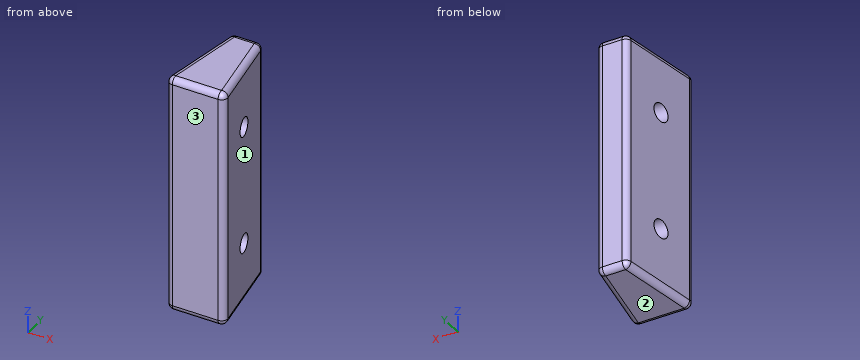
```python
from build123d import *

# Parameters (mm, degrees)
BOSS_EXTRUDE1_DEPTH     = 50.8
FILLET1_R               = 2.54
SKETCH4_R               = 3.96875
CUT_EXTRUDE1_DEPTH      = 13.241630529
CUT_EXTRUDE1_DEPTH_BACK = 13.241630529


with BuildPart() as part:
    # Sketch3 → Boss-Extrude1 (new body, symmetric)
    with BuildSketch(Plane.XY):
        Polygon((-12.7, 0), (12.7, 0), (6.35, 38.1), (-6.35, 38.1), align=None)
    extrude(amount=BOSS_EXTRUDE1_DEPTH, both=True)

    # Fillet1
    fillet1_edges = [part.edges().sort_by_distance(p)[0] for p in [
        (0, 0, 50.8),
        (9.525, 19.05, 50.8),
        (0, 38.1, 50.8),
        (9.525, 19.05, -50.8),
        (0, 0, -50.8),
        (-9.525, 19.05, -50.8),
        (0, 38.1, -50.8),
        (-9.525, 19.05, 50.8),
        (6.35, 38.1, 0),
        (12.7, 0, 0),
        (-12.7, 0, 0),
        (-6.35, 38.1, 0),
    ]]
    fillet(fillet1_edges, radius=FILLET1_R)

    # Sketch4 → Cut-Extrude1 (cut, two sides)
    with BuildSketch(Plane(origin=(0, 0, 0), x_dir=(0, 0, -1), z_dir=(1, 0, 0))) as cut_extrude1_sk:
        with Locations((-25.4, 19.05)):
            Circle(SKETCH4_R)
        with Locations((25.4, 19.05)):
            Circle(SKETCH4_R)
    extrude(amount=CUT_EXTRUDE1_DEPTH, mode=Mode.SUBTRACT)
    extrude(cut_extrude1_sk.sketch, amount=-CUT_EXTRUDE1_DEPTH_BACK, mode=Mode.SUBTRACT)


solid = part.part
```
For this review, take the finished solid that the model builds, in its own axes (mm). Face numbers are marked on the shaded views. Coordinates: 2 decimals unless noted, no trailing zeros. Loops run counter-clockwise (first coordinate to the right, second up) from the corner with the lowest first, then second, coordinate; pieces in that order, holes last.
1. Add section B-B, the plane z = 25.4. Give the boundary of the cut face in (x, y), then the cut area to 3 significant figures.
2. Mouldability with a two-part tool opening along Y and no side actions: class the marked faces 1, 2 and 3 as +Y half, -Y half, draft (parallel to the pull), parting line (faces both ways), or undercut.
3. Insertion check: P1, Ø6.5, axis at y = 19.05, z = 25.4, coming from the -X side; P2, Ø10, axis at y = 28, z = -35, coming from the -X side; P3, Ø9, axis at y = 19.05, z = -25.4, coming from the -X side (3 decimals). Each pin has a flat end and moves straight along its axis. Give the tip position at first contact, or say it passes through.
4. For line 1 (Z direction, x = 0.25, y = 19.05); line 2 (Y direction, x = 4.75, z = -25.5); line 3 (Y direction, x = 4.5, z = 12.5), list the stretches that pass through material, from the lowest coordinate up.
5. Add section C-C, the plane y = 19.05. Count the separate pieces of the cut face and the enclosed holes in it, then the cut area to 3 significant figures.
6. Add section A-A, the plane x = 3. Give the boundary of the cut face in (y, z), then the cut area to 3 significant figures.
Result:
1. outline: (-12.21, 2.96) arc R2.54 ccw to (-9.7, 0) - (9.7, 0) arc R2.54 ccw to (12.21, 2.96) - (10.19, 15.08) - (-10.19, 15.08) - close; (-8.86, 23.02) - (8.86, 23.02) - (6.7, 35.98) arc R2.54 ccw to (4.2, 38.1) - (-4.2, 38.1) arc R2.54 ccw to (-6.7, 35.98) - close
1. area: 569 mm2
2. face 1: +Y half
2. face 2: draft
2. face 3: -Y half
3. P1: passes through
3. P2: stops at x = -8.87
3. P3: stops at x = -10.275
4. line 1: z = -50.8 to -29.37, -21.43 to 21.43, 29.37 to 50.8
4. line 2: y = 0 to 15.08, 23.02 to 38.04
4. line 3: y = 0 to 38.08
5. separate pieces: 3
5. enclosed holes: 0
5. area: 1,630 mm2
6. outline: (0, -48.26) arc R2.54 ccw to (2.54, -50.8) - (35.56, -50.8) arc R2.54 ccw to (38.1, -48.26) - (38.1, 48.26) arc R2.54 ccw to (35.56, 50.8) - (2.54, 50.8) arc R2.54 ccw to (0, 48.26) - close; hole circle Ø7.94 at (19.05, -25.4); hole circle Ø7.94 at (19.05, 25.4)
6. area: 3,770 mm2
